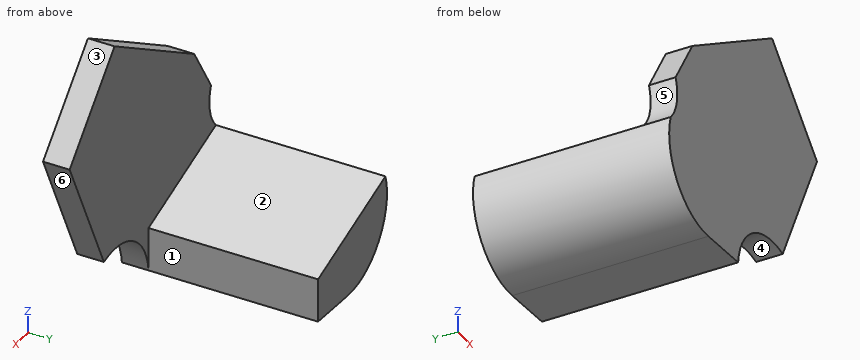
from build123d import *

# Parameters (mm, degrees)
BOSS_EXTRUDE1_DEPTH = 48.51400078
BOSS_EXTRUDE2_DEPTH = 7.62


with BuildPart() as part:
    # Sketch2 → Boss-Extrude1 (new body)
    with BuildSketch(Plane.XZ.offset(35.996799282)):
        with BuildLine():
            Line((-512.958981795, 54.074719549), (-477.784341144, 43.499133869))
            Line((-477.784341144, 43.499133869), (-477.784341144, 30.750375257))
            Line((-477.784341144, 30.750375257), (-493.297876549, 29.59254273))
            ThreePointArc((-493.297876549, 29.59254273), (-509.568926068, 36.66140776), (-512.958981795, 54.074719549))
        make_face()
    extrude(amount=BOSS_EXTRUDE1_DEPTH)

    # Sketch3 → Boss-Extrude2 (add)
    with BuildSketch(Plane.XZ.offset(84.510800062)):
        with BuildLine():
            Line((-460.055260418, 108.470724329), (-436.590512312, 84.974770196))
            Line((-436.590512312, 84.974770196), (-454.490518063, 46.803141976))
            ThreePointArc((-454.490518063, 46.803141976), (-469.864935435, 44.185661822), (-477.784341144, 30.750375257))
            Line((-477.784341144, 30.750375257), (-493.297876549, 29.59254273))
            ThreePointArc((-493.297876549, 29.59254273), (-509.568926068, 36.66140776), (-512.958981795, 54.074719549))
            ThreePointArc((-512.958981795, 54.074719549), (-509.76637554, 60.425881739), (-510.419261273, 67.504280999))
            Line((-510.419261273, 67.504280999), (-501.653310229, 82.024875489))
            Line((-501.653310229, 82.024875489), (-460.055260418, 108.470724329))
        make_face()
    extrude(amount=BOSS_EXTRUDE2_DEPTH)


solid = part.part
Check sheet for the modelled part. Datum: model origin and axes. Units: mm. Face numbers are marked on the shaded views. A direction names the side the tool comes from. Give positions to 0.01 mm unless a question says otherwise; leave off trailing zeros. Loops run counter-clockwise (first coordinate to the right, second up) from the corner with the lowest first, then second, coordinate; pieces in that order, holes last. Notation, with made-up numbers: M 5,52.25 L 49,52.25 A23 cw 49,73.25 Z; hole C 1,63.5 d3. An arc over 180 degrees is marked long. Use a Markdown table: item, result. Add a question column.
Q1. Scan lines: line 1 along Y through (x, z) = (-453.5, 91); line 2 along Z through (x, y) = (-498, -87); line 3 along Z through (x, y) = (-495, -83). Record each from-to range of solid material in increasing order. Write a range as [from, to].
Q2. Sectioned sample at B-B, the plane z = 73.5. Record the cut outline in (x, y).
Q3. Sectioned sample at D-D, the plane x = -486.5. Record the cut outline in (y, z).
Q4. Go/stop test with flat-tipped pins: pin 1 (4 mm diameter, centred on y = -52, z = 34.5, fed in from +X); pin 2 (12 mm diameter, centred on x = -476.5, y = -62, fed in from +Z); pin 3 (10 mm diameter, centred on x = -476.5, z = 98, fed in from +Y). Record where each tip stops, or that it passes through.
Q5. Sectioned sample at A-A, the plane x = -499.5. Record the cut outline in (y, z), then the cut area to 3 significant figures.
Q6. Mould release check, pull along X, two halves, no side actions. Record for the marked faces 4, 5 and 6: pulls with the +X half, pulls with the -X half, needs draft (parallel to the pull), parting line crosses it, or undercut.
Q7. Tool access check on the marked faces 1, 2 and 3. Record the directions out of +Z, -Z, +X, -X, +Y, -Y that give a thin tool (end or side, any length) a straight path to the whole face; none if there is none.
Q8. Sectioned sample at C-C, the plane y = -79. Record the cut outline in (x, z), then the cut area to 3 significant figures.
Verdict:
| question | item | result |
|---|---|---|
| 1 | line 1 | [-92.13, -84.51] |
| 1 | line 2 | [29.82, 84.35] |
| 1 | line 3 | [29.54, 48.68] |
| 2 | outline | M -506.8,-92.13 L -441.97,-92.13 L -441.97,-84.51 L -506.8,-84.51 Z |
| 3 | outline | M -92.13,30.1 L -36,30.1 L -36,46.12 L -84.51,46.12 L -84.51,91.66 L -92.13,91.66 Z |
| 4 | pin 1 | x = -477.78 |
| 4 | pin 2 | z = 44.92 |
| 4 | pin 3 | y = -84.51 |
| 5 | outline | M -92.13,30.15 L -36,30.15 L -36,50.03 L -84.51,50.03 L -84.51,83.39 L -92.13,83.39 Z |
| 5 | area | 1,370 mm^2 |
| 6 | face 4 | undercut |
| 6 | face 5 | pulls with the -X half |
| 6 | face 6 | pulls with the +X half |
| 7 | face 1 | +Z, -Z, +X, +Y |
| 7 | face 2 | +Z, +X, +Y |
| 7 | face 3 | +Z, +X, +Y, -Y |
| 8 | outline | M -512.96,54.07 A19.05 ccw -493.3,29.59 L -477.78,30.75 L -477.78,43.5 Z |
| 8 | area | 608 mm^2 |
